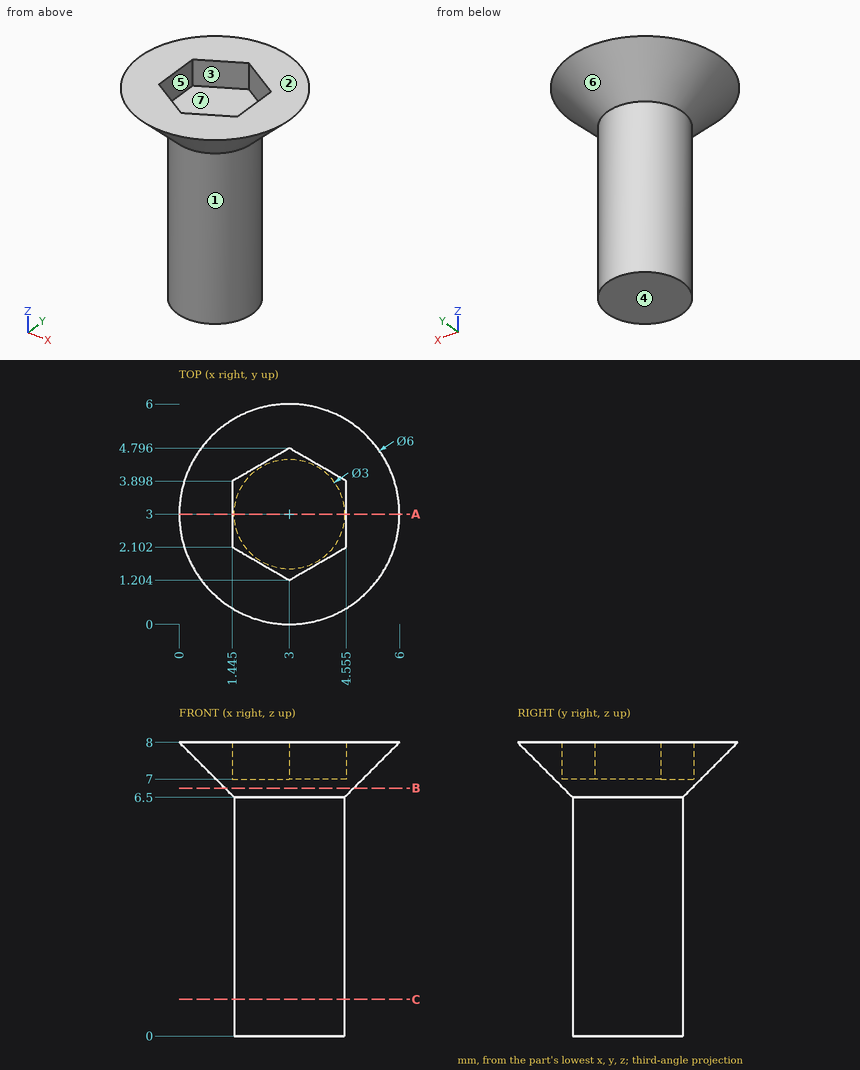
Source: three-view drawing plus pictorial views. Frame: mm from the lowest corner of the part. A direction names the side the tool comes from. Round coordinates to 2 decimals unless told otherwise and drop trailing zeros. Loops run counter-clockwise (first coordinate to the right, second up) from the corner with the lowest first, then second, coordinate; pieces in that order, holes last.
Q1. Section A-A, the plane y = 3. Return loops of the section in (x, z) (1 decimal).
Q2. First-contact query: P1, Ø0.5, axis at y = 2.5, z = 7.5, coming from the +X side; P2, Ø1, axis at y = 3, z = 3.5, coming from the -X side; P3, Ø0.5, axis at y = 2.5, z = 7.5, coming from the -X side. Flat tips, straight axial feed; report the tip coordinate or a pass-through.
Q3. Section B-B, the plane z = 6.75. Return loops of the section in (x, y).
Q4. Mould query, pull axis Y, two halves, no side actions, for the marked faces 4, 5, 6 and 7. Classes: pulls with the +Y half, pulls with the -Y half, needs draft (parallel to the pull), parting line crosses it, or undercut.
Q5. Ray query, line 1 (Z direction, x = 2.5, y = 2.65); line 2 (Y direction, x = 3.3, z = 7.5); line 3 (X direction, y = 4.6, z = 7.25) (1 decimal). Return the intervals inside material, ascending.
Q6. Section C-C, the plane z = 1. Return loops of the section in (x, y).
Q7. Access query for the marked faces 1, 2 and 3. Directions: +Z, -Z, +X, -X, +Y, -Y. A direction counts if a zero-diameter tool reaches every point of the face in a straight line with its end or side. Return the directions, or none.
Solutions:
1. outline: (0, 8) - (1.5, 6.5) - (1.5, 0) - (4.5, 0) - (4.5, 6.5) - (6, 8) - (4.6, 8) - (4.6, 7) - (1.4, 7) - (1.4, 8) - close
2. P1: stops at x = 5.71
2. P2: stops at x = 1.5
2. P3: stops at x = 0.29
3. outline: circle Ø3.5 at (3, 3)
4. face 4: needs draft
4. face 5: undercut
4. face 6: parting line crosses it
4. face 7: undercut
5. line 1: z = 0 to 7
5. line 2: y = 0.52 to 1.38, 4.62 to 5.48
5. line 3: x = 1.4 to 2.7, 3.3 to 4.6
6. outline: circle Ø3 at (3, 3)
7. face 1: -Z
7. face 2: +Z, +X, -X, +Y, -Y
7. face 3: +Z
